Build history of the part. All positions in model axes, mm. A direction names the side the tool comes from. Give positions to 0.01 mm unless a question says otherwise; leave off trailing zeros. Write each loop counter-clockwise with the first axis right and the second up, starting at its lowest first coordinate (ties: lowest second). Pieces come first, ordered by that corner, then holes.
from build123d import *

# Parameters (mm, degrees)
F0_R     = 6.35
F1_DEPTH = 19.05
F2_W     = 8.89
F2_H     = 25.4
F3_DEPTH = 25.4
F2_H_2   = 50.8
F4_DEPTH = 25.4


with BuildPart() as f1:
    # F0 (on Top) → F1 (new body)
    with BuildSketch(Plane.XY):
        Polygon((38.1, -12.7), (38.1, 12.7), (0, 12.7), (0, 38.1), (-38.1, 38.1), (-38.1, 12.7), (-38.1, -12.7), align=None)
        Circle(F0_R, mode=Mode.SUBTRACT)
        with Locations((-15.603517, 23.15443)):
            Circle(F0_R, mode=Mode.SUBTRACT)
    extrude(amount=F1_DEPTH)

    # F2 (on face) → F3 (join)
    with BuildSketch(Plane.XY.offset(19.05)):
        with Locations((33.655, 0)):
            Rectangle(F2_W, F2_H)
    extrude(amount=F3_DEPTH)

    # F2 (on face) → F4 (join)
    with BuildSketch(Plane.XY.offset(19.05)):
        with Locations((-33.655, 12.7)):
            Rectangle(F2_W, F2_H_2)
        with Locations((33.655, 0)):
            Rectangle(F2_W, F2_H)
    extrude(amount=F4_DEPTH)


solid = f1.part
1. Saw through at C-C on x = -10.5. Give the cut face in (y, z).
2. Drop flat-ended pins along their axis: pin 1 (6 mm diameter, centred on y = 23, z = 25.5, fed in from +X); pin 2 (5 mm diameter, centred on x = -22.5, y = 10.5, fed in from +Z). Give the stop position or say it passes through.
3. 3-axis set-ups, long thin cutter, end or side, ignore diameter. For faces 1 (the face through (34, 0, 44.45)), 2 (the face through (29.21, 0, 32)), 3 (the face through (0, 25, 9)): which of +Z, -Z, +X, -X, +Y, -Y reach the whole face in a straight line?
4. Mould opens along X. For faces 4 (the face through (-34, 13, 44.45)), 5 (the face through (-29.21, 12, 32)), 6 (the face through (38.1, 0, 22)), 7 (the face through (-1.38, -6.2, 9.39)) say: pulls with the +X half, pulls with the -X half, needs draft (parallel to the pull), parting line crosses it, or undercut.
5. Saw through at A-A on y = 0. Give the cut face in (x, z), plus the area to 3 significant figures.
6. Saw through at D-D on y = 8. Give the cut face in (x, z).
7. Drill centre lines: line 1 along X through (y, z) = (-1.5, 40); line 2 along X through (y, z) = (34, 25); line 3 along Z through (x, y) = (-20.5, 32.5). Where is each one in solid material? Low to high.
8. Saw through at B-B on z = 41. Give the cut face in (x, y), plus the area to 3 significant figures.
Outcome:
1. outline: (-12.7, 0) - (19.38, 0) - (19.38, 19.05) - (-12.7, 19.05) - close; (26.93, 0) - (38.1, 0) - (38.1, 19.05) - (26.93, 19.05) - close
2. pin 1: stops at x = -29.21
2. pin 2: stops at z = 19.05
3. face 1: +Z, +X, -X, +Y, -Y
3. face 2: +Z, +Y, -Y
3. face 3: +Z, -Z, +X, +Y
4. face 4: needs draft
4. face 5: undercut
4. face 6: pulls with the +X half
4. face 7: undercut
5. outline: (-38.1, 0) - (-6.35, 0) - (-6.35, 19.05) - (-29.21, 19.05) - (-29.21, 44.45) - (-38.1, 44.45) - close; (6.35, 0) - (38.1, 0) - (38.1, 44.45) - (29.21, 44.45) - (29.21, 19.05) - (6.35, 19.05) - close
5. area: 1,660 mm2
6. outline: (-38.1, 0) - (38.1, 0) - (38.1, 44.45) - (29.21, 44.45) - (29.21, 19.05) - (-29.21, 19.05) - (-29.21, 44.45) - (-38.1, 44.45) - close
7. line 1: x = -38.1 to -29.21, 29.21 to 38.1
7. line 2: x = -38.1 to -29.21
7. line 3: z = 0 to 19.05
8. outline: (-38.1, -12.7) - (-29.21, -12.7) - (-29.21, 38.1) - (-38.1, 38.1) - close; (29.21, -12.7) - (38.1, -12.7) - (38.1, 12.7) - (29.21, 12.7) - close
8. area: 677 mm2
